Geometry check sheet. Reference: the model listing, model coordinates, mm. A direction names the side the tool comes from. Coordinates: 2 decimals unless noted, no trailing zeros. Loops run counter-clockwise (first coordinate to the right, second up) from the corner with the lowest first, then second, coordinate; pieces in that order, holes last.
from build123d import *

# Parameters (mm, degrees)
SKETCH2_R           = 25.4
BOSS_EXTRUDE1_DEPTH = 152.4
BOSS_EXTRUDE2_DEPTH = 3.175


with BuildPart() as part:
    # Sketch2 → Boss-Extrude1 (new body)
    with BuildSketch(Plane(origin=(0, 0, 0), x_dir=(1, 0, 0), z_dir=(0, 1, 0))):
        with Locations(Location((0, 0, 0), (0, 0, 90))):
            Circle(SKETCH2_R)
    extrude(amount=BOSS_EXTRUDE1_DEPTH)

    # Sketch5 → 1 NPT Tapped Hole1 (revolve, cut)
    with BuildSketch(Plane(origin=(0, 0, 0), x_dir=(0, 0, -1), z_dir=(1, 0, 0))):
        Polygon((0, 0), (0, 59.506890972), (14.4907, 50.8), (14.4907, 16.764), (15.206530434, 16.764), (15.7298898, 0), align=None)
    revolve(axis=Axis((0, -6.35, 0), (0, 1, 0)), mode=Mode.SUBTRACT)



with BuildPart() as body_2:
    # Sketch7 → Boss-Extrude2 (new, symmetric)
    with BuildSketch(Plane.XY):
        Polygon((25.4, 152.4), (234.757779362, 76.2), (25.4, 0), (20.492740143, 0), (20.492740143, 152.4), align=None)
    extrude(amount=BOSS_EXTRUDE2_DEPTH, both=True)


with BuildPart() as part_1:
    add(part.part)

    add(body_2.part)  # Revolve1 merges body 2
    # Sketch8 → Revolve1 (revolve)
    with BuildSketch(Plane.XY):
        with BuildLine():
            Line((25.4, 152.4), (0, 152.4))
            Line((0, 152.4), (0, 236.290501198))
            ThreePointArc((0, 236.290501198), (43.825723586, 203.769361408), (25.4, 152.4))
        make_face()
    revolve(axis=Axis((0, 152.4, 0), (0, 1, 0)))


solid = part_1.part
(1) Sectioned sample at B-B on z = 34. Record the cut outline in (x, y), and give its area (3 significant figures).
Findings:
outline: circle Ø61.34 at (0, 190.5)
area: 2,960 mm2
(2) Gauge pin test, flat ends, axial feed: pin 1 Ø3 at (x, z) = (15, -23) entering from -Y; pin 2 Ø2 at (x, y) = (32.5, 139) entering from +Z (3 decimals); pin 3 Ø3 at (y, z) = (46, -7) entering from -X. Record the tip position at first contact, or that the pin passes through.
Findings:
pin 1: stops at y = 152.78
pin 2: stops at z = 3.175
pin 3: stops at x = -24.8
(3) Sectioned sample at D-D on x = 201. Record the cut outline in (y, z) (3 decimals), and give its area (3 significant figures).
Findings:
outline: (63.913, -3.175) - (88.487, -3.175) - (88.487, 3.175) - (63.913, 3.175) - close
area: 156 mm2
(4) Sectioned sample at C-C on y = 140. Record the cut outline in (x, z) (3 decimals).
Findings:
outline: (25.201, -3.175) - (59.469, -3.175) - (59.469, 3.175) - (25.201, 3.175) arc R25.4 ccw (long way) to start
(5) Access from +Z, -Z, +X, -X, +Y, -Y to the whole of each face (thin tool, end or side, straight path). Record for faces 1 (the flat face through (12, 0, -11)), 2 (the cylindrical face through (-25.377, 75.133, -1.072)).
Findings:
face 1: +Z, -Z, +X, -X, -Y
face 2: -Y
(6) Scan lines: L1, parallel to Z at x = 0, y = 38; L2, parallel to Z at x = 152, y = 63 (3 decimals); L3, parallel to Y at x = 7, z = -24. Record each from-to range of solid material in increasing order.
Findings:
L1: z = -25.4 to -14.49, 14.49 to 25.4
L2: z = -3.175 to 3.175
L3: y = 0 to 228.86
(7) Draft check along Z on faces 3 (the flat face through (108, 77, 3.175)), 4 (the cylindrical face through (-12.22, 33.54, -7.79)), 5 (the flat face through (108, 77, -3.175)), 6 (the conical face through (2.46, 57.99, 0.55)). Enter one of: +Z half, -Z half, draft (parallel to the pull), parting line (faces both ways), or undercut.
Findings:
face 3: +Z half
face 4: undercut
face 5: -Z half
face 6: undercut
(8) Sectioned sample at A-A on x = 35.5. Record the cut outline in (y, z) (3 decimals).
Findings:
outline: (3.676, -3.175) - (148.724, -3.175) - (148.724, 3.175) - (3.676, 3.175) - close; circle Ø57.845 at (190.5, 0)
